The model under review builds one solid part; all positions refer to its coordinate system, in mm. A direction names the side the tool comes from. Round coordinates to 2 decimals unless told otherwise and drop trailing zeros. Answer as a JSON object with one key per item and string values. Group by question number.
Item 1: The part is to be moulded in two halves that separate along X. For faces 1 (the face through (35.21, -4.88, 25.81)), 2 (the face through (30.34, -7.938, 10.22)), say which applies: +X half, -X half, draft (parallel to the pull), parting line (faces both ways), or undercut.
Item 2: Insertion check: P1, Ø2.5, axis at x = -0.34, z = 47.62, coming from the +Y side; P2, Ø2, axis at y = -4, z = 37.5, coming from the -X side; P3, Ø5, axis at x = -45.4, z = 14.39, coming from the -Y side; P4, Ø12, axis at x = -42, z = -43.5, coming from the -Y side. Each pin has a flat end and moves straight along its axis. Give the tip position at first contact, or say it passes through.
Item 3: To check wall thickness, follow line 1 (Z direction, x = 0, y = -4.5) (3 decimals); line 2 (Z direction, x = 10.5, y = -1); line 3 (Z direction, x = 12.5, y = -4.75). State the ranges of each line that lie inside material, in increasing order.
Item 4: Consider section A-A (z = 0). State how many separate pieces and enclosed holes the cut face has, and give its area (3 significant figures).
Item 5: Tool access review of faces 3 (the face through (25, -7.938, 33.3)), 4 (the face through (41.61, -4.876, -30.505)): name each direction out of +Z, -Z, +X, -X, +Y, -Y from which nothing blocks a thin tool from reaching the whole face with its end or side.
```python
from build123d import *

# Parameters (mm, degrees)
CSK_FOR_1_4_FLAT_HEAD_MACHINE_SCREW1_D           = 5.4102
CSK_FOR_1_4_FLAT_HEAD_MACHINE_SCREW1_CSINK_D     = 12.8778
CSK_FOR_1_4_FLAT_HEAD_MACHINE_SCREW1_CSINK_ANGLE = 82
SKETCH5_R                                        = 1.5875
RIVET_HOLES_DEPTH                                = 8.9375
CUT_EXTRUDE2_DEPTH                               = 6.2103
CHAMFER1_SIZE                                    = 0.2032


with BuildPart() as part:
    # Sketch1 → Revolve1 (revolve)
    with BuildSketch(Plane.XY):
        Polygon((31.623, 0), (31.623, -7.9375), (34.163, -7.9375), (34.163, -3.9497), (41.275, -3.9497), (41.275, -7.9375), (55.88, -7.9375), (55.88, 0), align=None)
    revolve(axis=Axis((0, 29.876386318, 0), (0, -1, 0)))

    # CSK for 1/4 Flat Head Machine Screw1 (through all)
    with Locations(Plane(origin=(0, 0, 0), x_dir=(-1, 0, 0), z_dir=(0, 1, 0))):
        with Locations((-47.625, 0), (-14.716934357, 45.294066589), (38.529434357, 27.99327264), (38.529434357, -27.99327264), (-14.716934357, -45.294066589)):
            CounterSinkHole(CSK_FOR_1_4_FLAT_HEAD_MACHINE_SCREW1_D / 2, CSK_FOR_1_4_FLAT_HEAD_MACHINE_SCREW1_CSINK_D / 2, counter_sink_angle=CSK_FOR_1_4_FLAT_HEAD_MACHINE_SCREW1_CSINK_ANGLE)

    # Sketch5 → Rivet Holes (cut, through all)
    with BuildSketch(Plane(origin=(0, 0, 0), x_dir=(1, 0, 0), z_dir=(0, 1, 0))):
        with Locations((-27.714283891, 38.730596347)):
            Circle(SKETCH5_R)
        with Locations((-0.343946691, 47.623757996)):
            Circle(SKETCH5_R)
        with Locations((28.270801327, 38.326262762)):
            Circle(SKETCH5_R)
        with Locations((45.1866, 15.043663299)):
            Circle(SKETCH5_R)
        with Locations((45.1866, -15.043663299)):
            Circle(SKETCH5_R)
        with Locations((28.270801327, -38.326262762)):
            Circle(SKETCH5_R)
        with Locations((-0.343946691, -47.623757996)):
            Circle(SKETCH5_R)
        with Locations((-27.714283891, -38.730596347)):
            Circle(SKETCH5_R)
        with Locations((-45.399170745, -14.389437815)):
            Circle(SKETCH5_R)
        with Locations((-45.399170745, 14.389437815)):
            Circle(SKETCH5_R)
    extrude(amount=-RIVET_HOLES_DEPTH, mode=Mode.SUBTRACT)

    # Sketch6 → Cut-Extrude2 (cut)
    with BuildSketch(Plane.XZ.offset(7.9375)):
        with BuildLine():
            ThreePointArc((48.95215, 16.297301907), (41.740220554, 30.32604536), (30.626701438, 41.520117993))
            ThreePointArc((30.626701438, 41.520117993), (25.076946097, 40.682162873), (25.914901216, 35.132407532))
            ThreePointArc((25.914901216, 35.132407532), (35.318648161, 25.66049992), (41.42105, 13.79002469))
            ThreePointArc((41.42105, 13.79002469), (46.440238608, 11.278113299), (48.95215, 16.297301907))
        make_face()
        with BuildLine():
            ThreePointArc((-0.372608915, 51.592404496), (-15.943345554, 49.068572138), (-30.023807548, 41.958146043))
            ThreePointArc((-30.023807548, 41.958146043), (-30.941833586, 36.42107269), (-25.404760233, 35.503046652))
            ThreePointArc((-25.404760233, 35.503046652), (-13.490523161, 41.51956104), (-0.315284467, 43.655111496))
            ThreePointArc((-0.315284467, 43.655111496), (3.624699809, 47.65242022), (-0.372608915, 51.592404496))
        make_face()
        with BuildLine():
            ThreePointArc((-49.182434974, 15.588557633), (-51.59375, 0), (-49.182434974, -15.588557633))
            ThreePointArc((-49.182434974, -15.588557633), (-44.200050927, -18.172702044), (-41.615906517, -13.190317997))
            ThreePointArc((-41.615906517, -13.190317997), (-43.65625, 0), (-41.615906517, 13.190317997))
            ThreePointArc((-41.615906517, 13.190317997), (-44.200050927, 18.172702044), (-49.182434974, 15.588557633))
        make_face()
        with BuildLine():
            ThreePointArc((-30.023807548, -41.958146043), (-15.943345554, -49.068572138), (-0.372608915, -51.592404496))
            ThreePointArc((-0.372608915, -51.592404496), (3.624699809, -47.65242022), (-0.315284467, -43.655111496))
            ThreePointArc((-0.315284467, -43.655111496), (-13.490523161, -41.51956104), (-25.404760233, -35.503046652))
            ThreePointArc((-25.404760233, -35.503046652), (-30.941833586, -36.42107269), (-30.023807548, -41.958146043))
        make_face()
        with BuildLine():
            ThreePointArc((30.626701438, -41.520117993), (41.740220554, -30.32604536), (48.95215, -16.297301907))
            ThreePointArc((48.95215, -16.297301907), (46.440238608, -11.278113299), (41.42105, -13.79002469))
            ThreePointArc((41.42105, -13.79002469), (35.318648161, -25.66049992), (25.914901216, -35.132407532))
            ThreePointArc((25.914901216, -35.132407532), (25.076946097, -40.682162873), (30.626701438, -41.520117993))
        make_face()
    extrude(amount=-CUT_EXTRUDE2_DEPTH, mode=Mode.SUBTRACT)

    # Chamfer1
    chamfer1_edges = [part.edges().sort_by_distance(p)[0] for p in [
        (-31.623, -7.9375, 0),
        (-55.88, -7.9375, 0),
        (-41.275, -7.9375, 0),
        (-34.163, -7.9375, 0),
    ]]
    chamfer(chamfer1_edges, length=CHAMFER1_SIZE)


solid = part.part
```
Geometry results:
{
 "1": {"face 1": "undercut", "face 2": "draft"},
 "2": {"P1": "passes through", "P2": "stops at x = -42.31", "P3": "stops at y = -1.73", "P4": "stops at y = -7.94"},
 "3": {"line 1": "z = -55.88 to -51.578, -43.67 to -41.275, -34.163 to -31.623, 31.623 to 34.163, 41.275 to 43.67, 51.578 to 55.88", "line 2": "z = -54.88 to -48.93, -41.66 to -29.83, 29.83 to 41.66, 48.93 to 54.88", "line 3": "z = -54.46 to -46.84, -43.74 to -39.34, -31.79 to -29.05, 29.05 to 31.79, 39.34 to 43.74, 46.84 to 54.46"},
 "4": {"separate pieces": "3", "enclosed holes": "0", "area": "220 mm^2"},
 "5": {"face 3": "+Z, -Z, +X, -X, -Y", "face 4": "-Y"}
}
